Part model, mm, in its own coordinate system. A direction names the side the tool comes from. Round coordinates to 2 decimals unless told otherwise and drop trailing zeros. Write each loop counter-clockwise with the first axis right and the second up, starting at its lowest first coordinate (ties: lowest second). Pieces come first, ordered by that corner, then holes. Notation, with made-up numbers: (-18, 56) -> (17, 56) arc R21 ccw to (17, 91) -> close; hole circle Ø6 at (-33.5, -33). An arc over 180 degrees is marked (long way). Use CSV: the item, a comma, the result in double quotes. Start each with the question number.
(1) Saw through at A-A (y = -36.5). Give the cut face in (x, z), plus the area to 3 significant figures.
(2) Probe line 1 (Z direction, x = -32.5, y = 11); line 2 (X direction, y = -282, z = -11); line 3 (Z direction, x = -7, y = 162). List the from-to ranges inside material, lowest first. Write a range as [from, to].
(3) Saw through at B-B (x = -49). Give the cut face in (y, z).
(4) Drop flat-ended pins along their axis: pin 1 (12 mm diameter, centred on x = -42, y = 3.5, fed in from +Z); pin 2 (1.6 mm diameter, centred on y = 353, z = -55.5, fed in from -X); pin 3 (14 mm diameter, centred on y = 43, z = -31, fed in from -X); pin 4 (13 mm diameter, centred on y = 0, z = -27, fed in from +X). Give the stop position or say it passes through.
(5) Saw through at C-C (z = -7). Give the cut face in (x, y).
(6) Which spindle directions (+Z, -Z, +X, -X, +Y, -Y) get a long thin tool onto all of the face, cutting with end or side? Do faces 1 (the flat face through (-31, 324, -56)), 2 (the flat face through (0, 5, -23)). Say none if no direction does.
```python
from build123d import *

# Parameters (mm, degrees)
SKETCH1_W                      = 2
SKETCH1_H                      = 710
BOSS_EXTRUDE1_DEPTH            = 2
BOSS_EXTRUDE3_DEPTH            = 2
CUT_EXTRUDE2_REACH             = 365.729
CUT_EXTRUDE2_DIRECTION_2_REACH = 365.729
BOSS_EXTRUDE5_DEPTH            = 355
BOSS_EXTRUDE5_DEPTH_BACK       = 355
SKETCH7_R                      = 5
CUT_EXTRUDE3_DEPTH             = 355
SKETCH8_R                      = 5
CUT_EXTRUDE4_DEPTH             = 355


with BuildPart() as part:
    # Sketch1 → Boss-Extrude1 (new body)
    with BuildSketch(Plane(origin=(0, 0, 0), x_dir=(0, 0, -1), z_dir=(1, 0, 0))):
        Polygon((0, 300), (0, 0), (55, 0), (55, 355), align=None)
        Polygon((0, 0), (0, -300), (55, -355), (55, 0), align=None)
        with Locations((56, 0)):
            Rectangle(SKETCH1_W, SKETCH1_H)
    extrude(amount=BOSS_EXTRUDE1_DEPTH)

    # Sketch2 → Boss-Extrude3 (add)
    with BuildSketch(Plane(origin=(0, 0, -57), x_dir=(-1, 0, 0), z_dir=(0, 0, -1))):
        Polygon((55, 300), (55, -300), (0, -355), (0, 355), align=None)
    extrude(amount=-BOSS_EXTRUDE3_DEPTH)

    # Sketch3 → Cut-Extrude2 (cut, up to next)
    with BuildSketch(Plane(origin=(0, 0, 0), x_dir=(-1, 0, 0), z_dir=(0, -1, 0)), mode=Mode.PRIVATE) as cut_extrude2_sk1:
        with BuildLine():
            Line((8, 57), (-2, 57))
            Line((-2, 57), (-2, 47))
            ThreePointArc((-2, 47), (0.928932188, 54.071067812), (8, 57))
        make_face()
    cut_extrude2_tool1 = extrude(cut_extrude2_sk1.sketch, amount=-CUT_EXTRUDE2_REACH, mode=Mode.PRIVATE) & part.part
    add(cut_extrude2_tool1.solids().sort_by_distance((-0.233679, 0, -54.766321))[0], mode=Mode.SUBTRACT)

    # Sketch3 → Cut-Extrude2 direction 2 (cut, up to next)
    with BuildSketch(Plane(origin=(0, 0, 0), x_dir=(-1, 0, 0), z_dir=(0, -1, 0)), mode=Mode.PRIVATE) as cut_extrude2_direction_2_sk1:
        with BuildLine():
            Line((8, 57), (-2, 57))
            Line((-2, 57), (-2, 47))
            ThreePointArc((-2, 47), (0.928932188, 54.071067812), (8, 57))
        make_face()
    cut_extrude2_direction_2_tool1 = extrude(cut_extrude2_direction_2_sk1.sketch, amount=CUT_EXTRUDE2_DIRECTION_2_REACH, mode=Mode.PRIVATE) & part.part
    add(cut_extrude2_direction_2_tool1.solids().sort_by_distance((-0.233679, 0, -54.766321))[0], mode=Mode.SUBTRACT)


with BuildPart() as cut_extrude2_piece_1:
    # of the separate pieces the step leaves, piece 1, a body of its own (cut_extrude2_pieces)
    add(part.part.solids().sort_by_distance((-8, -347, -57))[0])



with BuildPart() as cut_extrude2_piece_2:
    # of the separate pieces the step leaves, piece 2, a body of its own (cut_extrude2_pieces)
    add(part.part.solids().sort_by_distance((2, -347, -47))[0])


with BuildPart() as cut_extrude2_piece_1_1:
    add(cut_extrude2_piece_1.part)

    add(cut_extrude2_piece_2.part)  # Boss-Extrude5 merges Cut-Extrude2 piece 2
    # Sketch6 → Boss-Extrude5 (add, two sides: drawn at the far end of the back side and taken through both)
    with BuildSketch(Plane(origin=(0, 0, 0), x_dir=(-1, 0, 0), z_dir=(0, -1, 0)).offset(-BOSS_EXTRUDE5_DEPTH_BACK)):
        with BuildLine():
            Line((8, 55), (8, 57))
            ThreePointArc((8, 57), (0.928932188, 54.071067812), (-2, 47))
            Line((-2, 47), (0, 47))
            ThreePointArc((0, 47), (2.343145751, 52.656854249), (8, 55))
        make_face()
    extrude(amount=BOSS_EXTRUDE5_DEPTH + BOSS_EXTRUDE5_DEPTH_BACK)

    # Sketch7 → Cut-Extrude3 (cut)
    with BuildSketch(Plane(origin=(0, 0, -57), x_dir=(-1, 0, 0), z_dir=(0, 0, -1))):
        with Locations(Location((28, 0, 0), (0, 0, 90))):
            Circle(SKETCH7_R)
    extrude(amount=-CUT_EXTRUDE3_DEPTH, mode=Mode.SUBTRACT)

    # Sketch8 → Cut-Extrude4 (cut)
    with BuildSketch(Plane(origin=(2, 0, 0), x_dir=(0, 0, -1), z_dir=(1, 0, 0))):
        with Locations((27, 0)):
            Circle(SKETCH8_R)
    extrude(amount=-CUT_EXTRUDE4_DEPTH, mode=Mode.SUBTRACT)


solid = cut_extrude2_piece_1_1.part
```
Answers:
1,outline,"(-55, -57) -> (-8, -57) arc R10 ccw to (2, -47) -> (2, 0) -> (0, 0) -> (0, -47) arc R8 cw to (-8, -55) -> (-55, -55) -> close"
1,area,"216 mm²"
2,line 1,"z = [-57, -55]"
2,line 2,"x = [0, 2]"
2,line 3,"z = [-56.95, -54.94]"
3,outline,"(-306, -57) -> (306, -57) -> (306, -55) -> (-306, -55) -> close"
4,pin 1,"stops at z = -55"
4,pin 2,"stops at x = -8"
4,pin 3,"stops at x = 0"
4,pin 4,"stops at x = 2"
5,outline,"(0, -307) -> (2, -307) -> (2, 307) -> (0, 307) -> close"
6,face 1,"+Z, -Z, -X, +Y"
6,face 2,"+Z, -X, +Y, -Y"
